Verification items for the finished model (mm, model axes). A direction names the side the tool comes from. Coordinates: 2 decimals unless noted, no trailing zeros. Loops run counter-clockwise (first coordinate to the right, second up) from the corner with the lowest first, then second, coordinate; pieces in that order, holes last. Notation, with made-up numbers: (-28, -9.5) - (26, -9.5) arc R20 ccw to (26, 18.5) - close; hole circle Ø6 at (-13.5, 62.5). An arc over 180 degrees is marked (long way). Answer as CSV lines item,"result". Start each with the question number.
1. Set-up check for faces 5 (the flat face through (17, 4.15, 25)), 6 (the flat face through (-4.15, 17, 25)), 7 (the flat face through (16, 6.35, 25)): record each of +Z, -Z, +X, -X, +Y, -Y from which the full face is reachable in a straight line by a thin tool's end or side.
2. Material ranges on line 1 (Y direction, x = 14, z = 16.5); line 2 (Y direction, x = 0, z = 11.5); line 3 (Y direction, x = -9, z = 21.5), recorded low to high. Write a range as [from, to].
3. Gauge pin test, flat ends, axial feed: P1, Ø5, axis at x = -1.5, y = 13.5, coming from the -Z side; P2, Ø0.8, axis at y = 4.5, z = 13.5, coming from the -X side; P3, Ø1, axis at x = -2, z = 44.5, coming from the -Y side; P4, Ø1.1, axis at y = -19.5, z = 26, coming from the -X side. Record the tip position at first contact, or that the pin passes through.
4. Release check for a two-part mould opening along Y. For faces 1 (the flat face through (5.85, 0, 25)), 2 (the flat face through (15, 10.3, 25)), 3 (the cylindrical face through (-19.36, 19.32, 24.65)), 4 (the flat face through (4.15, -17, 25)) record: pulls with the +Y half, pulls with the -Y half, needs draft (parallel to the pull), parting line crosses it, or undercut.
5. Cross-section at B-B (y = 0). Enter the section's corners in (x, z), plus the area to 3 significant figures.
6. Cross-section at D-D (z = 26.5). State how many separate pieces and enclosed holes the cut face has, plus the area to 3 significant figures.
7. Cross-section at A-A (y = -13.5). Enter the section's corners in (x, z).
```python
from build123d import *

# Parameters (mm, degrees)
SKETCH1_R           = 3.4
BOSS_EXTRUDE1_DEPTH = 713
SKETCH2_W           = 40
SKETCH2_H           = 113
CUT_EXTRUDE1_DEPTH  = 715.401147815
SKETCH3_W           = 40
SKETCH3_H           = 550
CUT_EXTRUDE2_DEPTH  = 602.66435826


with BuildPart() as part:
    # Sketch1 → Boss-Extrude1 (new body)
    with BuildSketch(Plane.XY):
        with BuildLine():
            Line((20, 17.75), (20, 5.15))
            Line((20, 5.15), (19, 5.15))
            Line((19, 5.15), (19, 4.15))
            Line((19, 4.15), (15.4, 4.15))
            Line((15.4, 4.15), (15.4, 6.35))
            Line((15.4, 6.35), (16.95, 6.35))
            ThreePointArc((16.95, 6.35), (17.833883476, 6.716116524), (18.2, 7.6))
            Line((18.2, 7.6), (18.2, 9.3))
            ThreePointArc((18.2, 9.3), (17.907106781, 10.007106781), (17.2, 10.3))
            Line((17.2, 10.3), (12.03669957, 10.3))
            ThreePointArc((12.03669957, 10.3), (11.73040037, 10.239040459), (11.470780817, 10.065452001))
            Line((11.470780817, 10.065452001), (6.084081247, 4.674305984))
            ThreePointArc((6.084081247, 4.674305984), (5.910833239, 4.414848262), (5.85, 4.108853983))
            Line((5.85, 4.108853983), (5.85, -4.108853983))
            ThreePointArc((5.85, -4.108853983), (5.910833239, -4.414848262), (6.084081247, -4.674305984))
            Line((6.084081247, -4.674305984), (11.470780817, -10.065452001))
            ThreePointArc((11.470780817, -10.065452001), (11.73040037, -10.239040459), (12.03669957, -10.3))
            Line((12.03669957, -10.3), (17.2, -10.3))
            ThreePointArc((17.2, -10.3), (17.907106781, -10.007106781), (18.2, -9.3))
            Line((18.2, -9.3), (18.2, -7.6))
            ThreePointArc((18.2, -7.6), (17.833883476, -6.716116524), (16.95, -6.35))
            Line((16.95, -6.35), (15.4, -6.35))
            Line((15.4, -6.35), (15.4, -4.15))
            Line((15.4, -4.15), (19, -4.15))
            Line((19, -4.15), (19, -5.15))
            Line((19, -5.15), (20, -5.15))
            Line((20, -5.15), (20, -17.75))
            ThreePointArc((20, -17.75), (19.340990258, -19.340990258), (17.75, -20))
            Line((17.75, -20), (5.15, -20))
            Line((5.15, -20), (5.15, -19))
            Line((5.15, -19), (4.15, -19))
            Line((4.15, -19), (4.15, -15.4))
            Line((4.15, -15.4), (6.35, -15.4))
            Line((6.35, -15.4), (6.35, -16.95))
            ThreePointArc((6.35, -16.95), (6.716116524, -17.833883476), (7.6, -18.2))
            Line((7.6, -18.2), (9.3, -18.2))
            ThreePointArc((9.3, -18.2), (10.007106781, -17.907106781), (10.3, -17.2))
            Line((10.3, -17.2), (10.3, -12.054477022))
            ThreePointArc((10.3, -12.054477022), (10.239166761, -11.748482743), (10.065918753, -11.489025021))
            Line((10.065918753, -11.489025021), (4.665899173, -6.084547999))
            ThreePointArc((4.665899173, -6.084547999), (4.406279619, -5.910959541), (4.09998042, -5.85))
            Line((4.09998042, -5.85), (-4.09998042, -5.85))
            ThreePointArc((-4.09998042, -5.85), (-4.406279619, -5.910959541), (-4.665899173, -6.084547999))
            Line((-4.665899173, -6.084547999), (-10.065918753, -11.489025021))
            ThreePointArc((-10.065918753, -11.489025021), (-10.239166761, -11.748482743), (-10.3, -12.054477022))
            Line((-10.3, -12.054477022), (-10.3, -17.2))
            ThreePointArc((-10.3, -17.2), (-10.007106781, -17.907106781), (-9.3, -18.2))
            Line((-9.3, -18.2), (-7.6, -18.2))
            ThreePointArc((-7.6, -18.2), (-6.716116524, -17.833883476), (-6.35, -16.95))
            Line((-6.35, -16.95), (-6.35, -15.4))
            Line((-6.35, -15.4), (-4.15, -15.4))
            Line((-4.15, -15.4), (-4.15, -19))
            Line((-4.15, -19), (-5.15, -19))
            Line((-5.15, -19), (-5.15, -20))
            Line((-5.15, -20), (-17.75, -20))
            ThreePointArc((-17.75, -20), (-19.340990258, -19.340990258), (-20, -17.75))
            Line((-20, -17.75), (-20, -5.15))
            Line((-20, -5.15), (-19, -5.15))
            Line((-19, -5.15), (-19, -4.15))
            Line((-19, -4.15), (-15.4, -4.15))
            Line((-15.4, -4.15), (-15.4, -6.35))
            Line((-15.4, -6.35), (-16.95, -6.35))
            ThreePointArc((-16.95, -6.35), (-17.833883476, -6.716116524), (-18.2, -7.6))
            Line((-18.2, -7.6), (-18.2, -9.3))
            ThreePointArc((-18.2, -9.3), (-17.907106781, -10.007106781), (-17.2, -10.3))
            Line((-17.2, -10.3), (-12.03669957, -10.3))
            ThreePointArc((-12.03669957, -10.3), (-11.73040037, -10.239040459), (-11.470780817, -10.065452001))
            Line((-11.470780817, -10.065452001), (-6.084081247, -4.674305984))
            ThreePointArc((-6.084081247, -4.674305984), (-5.910833239, -4.414848262), (-5.85, -4.108853983))
            Line((-5.85, -4.108853983), (-5.85, 4.108853983))
            ThreePointArc((-5.85, 4.108853983), (-5.910833239, 4.414848262), (-6.084081247, 4.674305984))
            Line((-6.084081247, 4.674305984), (-11.470780817, 10.065452001))
            ThreePointArc((-11.470780817, 10.065452001), (-11.73040037, 10.239040459), (-12.03669957, 10.3))
            Line((-12.03669957, 10.3), (-17.2, 10.3))
            ThreePointArc((-17.2, 10.3), (-17.907106781, 10.007106781), (-18.2, 9.3))
            Line((-18.2, 9.3), (-18.2, 7.6))
            ThreePointArc((-18.2, 7.6), (-17.833883476, 6.716116524), (-16.95, 6.35))
            Line((-16.95, 6.35), (-15.4, 6.35))
            Line((-15.4, 6.35), (-15.4, 4.15))
            Line((-15.4, 4.15), (-19, 4.15))
            Line((-19, 4.15), (-19, 5.15))
            Line((-19, 5.15), (-20, 5.15))
            Line((-20, 5.15), (-20, 17.75))
            ThreePointArc((-20, 17.75), (-19.340990258, 19.340990258), (-17.75, 20))
            Line((-17.75, 20), (-5.15, 20))
            Line((-5.15, 20), (-5.15, 19))
            Line((-5.15, 19), (-4.15, 19))
            Line((-4.15, 19), (-4.15, 15.4))
            Line((-4.15, 15.4), (-6.35, 15.4))
            Line((-6.35, 15.4), (-6.35, 16.95))
            ThreePointArc((-6.35, 16.95), (-6.716116524, 17.833883476), (-7.6, 18.2))
            Line((-7.6, 18.2), (-9.3, 18.2))
            ThreePointArc((-9.3, 18.2), (-10.007106781, 17.907106781), (-10.3, 17.2))
            Line((-10.3, 17.2), (-10.3, 12.054477022))
            ThreePointArc((-10.3, 12.054477022), (-10.239166761, 11.748482743), (-10.065918753, 11.489025021))
            Line((-10.065918753, 11.489025021), (-4.665899173, 6.084547999))
            ThreePointArc((-4.665899173, 6.084547999), (-4.406279619, 5.910959541), (-4.09998042, 5.85))
            Line((-4.09998042, 5.85), (4.09998042, 5.85))
            ThreePointArc((4.09998042, 5.85), (4.406279619, 5.910959541), (4.665899173, 6.084547999))
            Line((4.665899173, 6.084547999), (10.065918753, 11.489025021))
            ThreePointArc((10.065918753, 11.489025021), (10.239166761, 11.748482743), (10.3, 12.054477022))
            Line((10.3, 12.054477022), (10.3, 17.2))
            ThreePointArc((10.3, 17.2), (10.007106781, 17.907106781), (9.3, 18.2))
            Line((9.3, 18.2), (7.6, 18.2))
            ThreePointArc((7.6, 18.2), (6.716116524, 17.833883476), (6.35, 16.95))
            Line((6.35, 16.95), (6.35, 15.4))
            Line((6.35, 15.4), (4.15, 15.4))
            Line((4.15, 15.4), (4.15, 19))
            Line((4.15, 19), (5.15, 19))
            Line((5.15, 19), (5.15, 20))
            Line((5.15, 20), (17.75, 20))
            ThreePointArc((17.75, 20), (19.340990258, 19.340990258), (20, 17.75))
        make_face()
        with Locations(Location((0, 0, 0), (0, 0, 180))):
            Circle(SKETCH1_R, mode=Mode.SUBTRACT)
        with BuildLine():
            Line((18.6, 16.35), (18.6, 12.2))
            ThreePointArc((18.6, 12.2), (18.365685425, 11.634314575), (17.8, 11.4))
            Line((17.8, 11.4), (12.2, 11.4))
            ThreePointArc((12.2, 11.4), (11.634314575, 11.634314575), (11.4, 12.2))
            Line((11.4, 12.2), (11.4, 17.8))
            ThreePointArc((11.4, 17.8), (11.634314575, 18.365685425), (12.2, 18.6))
            Line((12.2, 18.6), (16.35, 18.6))
            ThreePointArc((16.35, 18.6), (17.940990258, 17.940990258), (18.6, 16.35))
        make_face(mode=Mode.SUBTRACT)
        with BuildLine():
            Line((-12.2, 18.6), (-16.35, 18.6))
            ThreePointArc((-16.35, 18.6), (-17.940990258, 17.940990258), (-18.6, 16.35))
            Line((-18.6, 16.35), (-18.6, 12.2))
            ThreePointArc((-18.6, 12.2), (-18.365685425, 11.634314575), (-17.8, 11.4))
            Line((-17.8, 11.4), (-12.2, 11.4))
            ThreePointArc((-12.2, 11.4), (-11.634314575, 11.634314575), (-11.4, 12.2))
            Line((-11.4, 12.2), (-11.4, 17.8))
            ThreePointArc((-11.4, 17.8), (-11.634314575, 18.365685425), (-12.2, 18.6))
        make_face(mode=Mode.SUBTRACT)
        with BuildLine():
            Line((-18.6, -16.35), (-18.6, -12.2))
            ThreePointArc((-18.6, -12.2), (-18.365685425, -11.634314575), (-17.8, -11.4))
            Line((-17.8, -11.4), (-12.2, -11.4))
            ThreePointArc((-12.2, -11.4), (-11.634314575, -11.634314575), (-11.4, -12.2))
            Line((-11.4, -12.2), (-11.4, -17.8))
            ThreePointArc((-11.4, -17.8), (-11.634314575, -18.365685425), (-12.2, -18.6))
            Line((-12.2, -18.6), (-16.35, -18.6))
            ThreePointArc((-16.35, -18.6), (-17.940990258, -17.940990258), (-18.6, -16.35))
        make_face(mode=Mode.SUBTRACT)
        with BuildLine():
            Line((12.2, -18.6), (16.35, -18.6))
            ThreePointArc((16.35, -18.6), (17.940990258, -17.940990258), (18.6, -16.35))
            Line((18.6, -16.35), (18.6, -12.2))
            ThreePointArc((18.6, -12.2), (18.365685425, -11.634314575), (17.8, -11.4))
            Line((17.8, -11.4), (12.2, -11.4))
            ThreePointArc((12.2, -11.4), (11.634314575, -11.634314575), (11.4, -12.2))
            Line((11.4, -12.2), (11.4, -17.8))
            ThreePointArc((11.4, -17.8), (11.634314575, -18.365685425), (12.2, -18.6))
        make_face(mode=Mode.SUBTRACT)
    extrude(amount=BOSS_EXTRUDE1_DEPTH)

    # Sketch2 → Cut-Extrude1 (cut, through all)
    with BuildSketch(Plane(origin=(0, 20, 0), x_dir=(1, 0, 0), z_dir=(0, 1, 0))):
        with Locations((0, -656.5)):
            Rectangle(SKETCH2_W, SKETCH2_H)
    extrude(amount=-CUT_EXTRUDE1_DEPTH, mode=Mode.SUBTRACT)

    # Sketch3 → Cut-Extrude2 (cut, through all)
    with BuildSketch(Plane(origin=(0, 20, 0), x_dir=(1, 0, 0), z_dir=(0, 1, 0))):
        with Locations((0, -325)):
            Rectangle(SKETCH3_W, SKETCH3_H)
    extrude(amount=-CUT_EXTRUDE2_DEPTH, mode=Mode.SUBTRACT)


solid = part.part
```
Values follow:
1,face 5,"+Z, -Z, +X"
1,face 6,"+Z, -Z, +Y"
1,face 7,"+Z, -Z"
2,line 1,"y = [-20, -18.6], [-11.4, -10.3], [10.3, 11.4], [18.6, 20]"
2,line 2,"y = [-5.85, -3.4], [3.4, 5.85]"
2,line 3,"y = [-20, -18.2], [-10.42, -7.59], [7.59, 10.42], [18.2, 20]"
3,P1,"passes through"
3,P2,"stops at x = -19"
3,P3,"stops at y = -5.85"
3,P4,"stops at x = -19.65"
4,face 1,"undercut"
4,face 2,"undercut"
4,face 3,"pulls with the +Y half"
4,face 4,"needs draft"
5,outline,"(-5.85, 0) - (-3.4, 0) - (-3.4, 50) - (-5.85, 50) - close; (3.4, 0) - (5.85, 0) - (5.85, 50) - (3.4, 50) - close"
5,area,"245 mm²"
6,separate pieces,"1"
6,enclosed holes,"5"
6,area,"464 mm²"
7,outline,"(-20, 0) - (-18.6, 0) - (-18.6, 50) - (-20, 50) - close; (-11.4, 0) - (-10.3, 0) - (-10.3, 50) - (-11.4, 50) - close; (10.3, 0) - (11.4, 0) - (11.4, 50) - (10.3, 50) - close; (18.6, 0) - (20, 0) - (20, 50) - (18.6, 50) - close"
